```python
from build123d import *

# Parameters (mm, degrees)
F0_W      = 150
F0_H      = 150
F1_DEPTH  = 12.5
F3_DEPTH  = 50
F5_R      = 22.5
F6_DEPTH  = 90
F8_R      = 22.5
F9_DEPTH  = 90
F11_DEPTH = 9.5
F13_DEPTH = 7.5
F15_DEPTH = 3.2
F16_R     = 2
F17_DEPTH = 6.4
F18_R     = 10
F19_DEPTH = 160.001
F20_R     = 10
F21_DEPTH = 160.001


with BuildPart() as f1:
    # F0 (on Top) → F1 (new body)
    with BuildSketch(Plane.XY):
        Rectangle(F0_W, F0_H)
    extrude(amount=F1_DEPTH)

    # F2 (on face) → F3 (join)
    with BuildSketch(Plane.XY.offset(12.5)):
        with BuildLine():
            Line((-35, -15), (-35, -75))
            Line((-35, -75), (-25, -75))
            Line((-25, -75), (-25, -23.9734782516))
            ThreePointArc((-25, -23.9734782516), (7.0710678119, -7.0710678119), (23.9734782516, 25))
            Line((23.9734782516, 25), (75, 25))
            Line((75, 25), (75, 35))
            Line((75, 35), (15, 35))
            ThreePointArc((15, 35), (0, 0), (-35, -15))
        make_face()
    extrude(amount=F3_DEPTH)

    # F5 (on offset) → F6 (join)
    with BuildSketch(Plane.XZ.offset(85)):
        with Locations((-30, 62.5)):
            Circle(F5_R)
    extrude(amount=-F6_DEPTH)

    # F8 (on offset) → F9 (join)
    with BuildSketch(Plane.YZ.offset(85)):
        with Locations((30, 62.5)):
            Circle(F8_R)
    extrude(amount=-F9_DEPTH)

    # F10 (on face) → F11 (join)
    with BuildSketch(Plane.XY.offset(12.5)):
        with BuildLine():
            Line((25, -75), (75, -75))
            Line((75, -75), (75, -25))
            Line((75, -25), (30, -25))
            ThreePointArc((30, -25), (26.4644660941, -26.4644660941), (25, -30))
            Line((25, -30), (25, -75))
        make_face()
    extrude(amount=F11_DEPTH)

    # F12 (on face) → F13 (join)
    with BuildSketch(Plane.XY.offset(12.5)):
        with BuildLine():
            Line((27.6014252577, 20.5), (70.5, 20.5))
            Line((70.5, 20.5), (70.5, -25))
            Line((70.5, -25), (75, -25))
            Line((75, -25), (75, 25))
            Line((75, 25), (23.9734782516, 25))
            ThreePointArc((23.9734782516, 25), (7.0710678119, -7.0710678119), (-25, -23.9734782516))
            Line((-25, -23.9734782516), (-25, -75))
            Line((-25, -75), (25, -75))
            Line((25, -75), (25, -70.5))
            Line((25, -70.5), (-20.5, -70.5))
            Line((-20.5, -70.5), (-20.5, -27.6014252577))
            ThreePointArc((-20.5, -27.6014252577), (10.2530483272, -10.2530483272), (27.6014252577, 20.5))
        make_face()
    extrude(amount=F13_DEPTH)

    # F14 (on face) → F15 (cut)
    with BuildSketch(Plane.XY.offset(22)):
        Polygon((52.0207259422, -46.5), (47.9792740578, -46.5), (45.9585481157, -50), (47.9792740578, -53.5), (52.0207259422, -53.5), (54.0414518843, -50), align=None)
    extrude(amount=-F15_DEPTH, mode=Mode.SUBTRACT)

    # F16 (on face) → F17 (cut)
    with BuildSketch(Plane.XY.offset(18.8)):
        with Locations((50, -50)):
            Circle(F16_R)
    extrude(amount=-F17_DEPTH, mode=Mode.SUBTRACT)

    # F18 (on face) → F19 (cut, through all)
    with BuildSketch(Plane.XZ.offset(85)):
        with Locations((-30, 62.5)):
            Circle(F18_R)
    extrude(amount=-F19_DEPTH, mode=Mode.SUBTRACT)

    # F20 (on face) → F21 (cut, through all)
    with BuildSketch(Plane.YZ.offset(85)):
        with Locations((30, 62.5)):
            Circle(F20_R)
    extrude(amount=-F21_DEPTH, mode=Mode.SUBTRACT)


solid = f1.part
```
Input: part model. Units: mm. Frame: model coordinates. A direction names the side the tool comes from. Give positions to 0.01 mm unless a question says otherwise; leave off trailing zeros. Order: outer loops, then holes, each group sorted by start corner. A loop starts at its lowest first (then second) coordinate and runs counter-clockwise, first axis right, second up.
1. Section C-C on x = 50. Return the cut outline in (y, z).
Derived:
outline: (-75, 0) - (75, 0) - (75, 12.5) - (35, 12.5) - (35, 40.56) arc R22.5 ccw (long way) to (25, 40.56) - (25, 20) - (20.5, 20) - (20.5, 12.5) - (-25, 12.5) - (-25, 22) - (-46.5, 22) - (-46.5, 18.8) - (-48, 18.8) - (-48, 12.4) - (-52, 12.4) - (-52, 18.8) - (-53.5, 18.8) - (-53.5, 22) - (-75, 22) - close; hole circle Ø20 at (30, 62.5)
2. Section B-B on y = -44. Return the cut outline in (x, z), and give its area (3 significant figures).
Derived:
outline: (-75, 0) - (75, 0) - (75, 22) - (25, 22) - (25, 12.5) - (-20.5, 12.5) - (-20.5, 20) - (-25, 20) - (-25, 40.56) arc R22.5 ccw (long way) to (-35, 40.56) - (-35, 12.5) - (-75, 12.5) - close; hole circle Ø20 at (-30, 62.5)
area: 3,940 mm2
3. Section A-A on z = 59. Return the cut outline in (x, y), and give its area (3 significant figures).
Derived:
outline: (-52.23, -85) - (-39.37, -85) - (-39.37, 5) - (-52.23, 5) - close; (-20.63, -85) - (-7.77, -85) - (-7.77, -18) arc R61.27 ccw to (18, 7.77) - (85, 7.77) - (85, 20.63) - (-5, 20.63) - (-5, 7.77) - (6.38, 7.77) arc R51.27 cw to (-7.77, -6.38) - (-7.77, 5) - (-20.63, 5) - close; (-5, 39.37) - (85, 39.37) - (85, 52.23) - (-5, 52.23) - close
area: 4,920 mm2
4. Reachability of faces 1 (the flat face through (53, -25, 17)), 2 (the cylindrical face through (6.71, -7.43, 36.23)), 3 (the flat face through (49, 20.5, 16)) from +Z, -Z, +X, -X, +Y, -Y: full face, straight path, thin tool, end or side. Return the list, or none.
Derived:
face 1: +Z
face 2: +X, -Y
face 3: none
5. Section D-D on y = 47. Return the cut outline in (x, z), and give its area (3 significant figures).
Derived:
outline: (-75, 0) - (75, 0) - (75, 12.5) - (-75, 12.5) - close; (-5, 47.76) - (85, 47.76) - (85, 77.24) - (-5, 77.24) - close
area: 4,530 mm2
6. Material intervals for L1, parallel to Y at x = 50, z = 16.75; L2, parallel to Z at x = 55, y = 30; L3, parallel to Y at x = 53, z = 62, sorted ascending.
Derived:
L1: y = -75 to -52, -48 to -25, 20.5 to 35
L2: z = 0 to 52.5, 72.5 to 85
L3: y = 7.51 to 20.01, 39.99 to 52.49
7. Mould query, pull axis Y, two halves, no side actions, for faces 4 (the flat face through (44, -50, 22)), 5 (the flat face through (-1, -75, 11)), 6 (the flat face through (10, -10, 20)). Classes: released by +Y, released by -Y, zero draft, split by the parting line, or undercut.
Derived:
face 4: zero draft
face 5: released by -Y
face 6: undercut
8. Pin query (flat end, axial travel): pin 1 (7.5 mm diameter, centred on x = 46.5, z = 18.5, fed in from +Y); pin 2 (12 mm diameter, centred on x = 25.5, y = -28.5, fed in from +Z); pin 3 (8 mm diameter, centred on x = 46.5, z = 16, fed in from -Y). Return the tip coordinate at first contact, or that it passes through.
Derived:
pin 1: stops at y = 35
pin 2: stops at z = 22
pin 3: stops at y = -75
